from build123d import *

# Parameters (mm, degrees)
F0_R     = 1.5
F0_R_2   = 3
F1_DEPTH = 2


with BuildPart() as f1:
    # F0 (on Top) → F1 (new body)
    with BuildSketch(Plane.XY):
        with BuildLine():
            Line((-31.964893, 11.673815), (-28.487817, 11.673815))
            Line((-28.487817, 11.673815), (-28.487817, 7.80591))
            ThreePointArc((-28.487817, 7.80591), (-24.73358, 5.237709), (-20.981651, 7.80928))
            Line((-20.981651, 7.80928), (-20.981651, 11.050785))
            Line((-20.981651, 11.050785), (-15.487817, 11.050785))
            ThreePointArc((-15.487817, 11.050785), (-13.62272, 14.450413), (-15.487817, 17.850041))
            Line((-15.487817, 17.850041), (-15.487817, 21.423815))
            Line((-15.487817, 21.423815), (-21.987817, 21.423815))
            ThreePointArc((-21.987817, 21.423815), (-24.399065, 23.705329), (-27.288638, 22.071378))
            Line((-27.288638, 22.071378), (-31.889195, 17.850041))
            ThreePointArc((-31.889195, 17.850041), (-33.985999, 17.050288), (-34.987817, 15.042166))
            Line((-34.987817, 15.042166), (-34.987817, 14.481326))
            ThreePointArc((-34.987817, 14.481326), (-34.01389, 12.498791), (-31.964893, 11.673815))
        make_face()
        with Locations((-24.737817, 8.548815)):
            Circle(F0_R, mode=Mode.SUBTRACT)
        with Locations((-32.562817, 14.673815)):
            Circle(F0_R, mode=Mode.SUBTRACT)
        with Locations((-24.737817, 14.673815)):
            Circle(F0_R_2, mode=Mode.SUBTRACT)
        with Locations((-24.737817, 20.798815)):
            Circle(F0_R, mode=Mode.SUBTRACT)
        with Locations((-16.912817, 14.673815)):
            Circle(F0_R, mode=Mode.SUBTRACT)
    extrude(amount=F1_DEPTH)


solid = f1.part
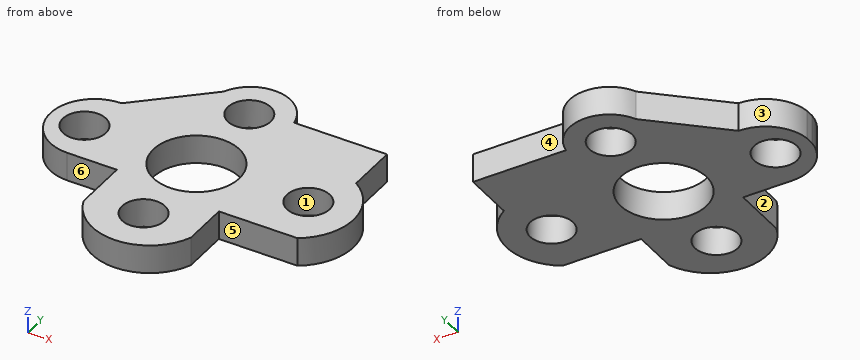
Here's how the part is built. I have some questions about the finished solid (model axes, mm). Face numbers are marked on the shaded views. A direction names the side the tool comes from. Give positions to 0.01 mm unless a question says otherwise; leave off trailing zeros. Loops run counter-clockwise (first coordinate to the right, second up) from the corner with the lowest first, then second, coordinate; pieces in that order, holes last. Notation, with made-up numbers: (84.25, -26) -> (141.25, -26) arc R10 ccw to (141.25, -18) -> close; hole circle Ø5 at (10, 27.25). An arc over 180 degrees is marked (long way). Answer as a JSON object with one key per item and string values. Group by question number.
Item 1: Imagine slicing it at B-B on x = -25.25. Write out the boundary of the cut face in (y, z).
Item 2: Imagine slicing it at D-D on y = 20.25. Write out the boundary of the cut face in (x, z).
Item 3: Imagine slicing it at A-A on y = 15.75. Write out the boundary of the cut face in (x, z), then the cut area to 3 significant figures.
Item 4: Imagine slicing it at C-C on x = -23. Write out the boundary of the cut face in (y, z).
Item 5: I need wall thicknesses on L1, parallel to Y at x = -25, z = 1.2; L2, parallel to X at y = 15.75, z = 0.4; L3, parallel to Y at x = -17.5, z = 0.5. Which ranges of each line are inside material? Lowest first, please.
Item 6: On a 3-axis mill with a long thin cutter (end or side, diameter ignored), from which of +Z, -Z, +X, -X, +Y, -Y can I reach the whole of each face in a straight line? I mean the marked faces 4, 5 and 6. Say none if no direction works.
Item 7: Will these pins go through, and if not, where does the flat tip stop? pin 1 (1 mm diameter, centred on y = 18.5, z = 0.5, fed in from -X); pin 2 (0.6 mm diameter, centred on y = 10.5, z = 1.5, fed in from -X); pin 3 (3.5 mm diameter, centred on x = -24.74, y = 14.67, fed in from +Z); pin 4 (0.6 mm diameter, centred on x = -17, z = 1, fed in from -Y).
Item 8: Thinking about a two-plate mould opening in Y: for the marked faces 1, 2 and 3, which applies, pulls with the +Y half, pulls with the -Y half, needs draft (parallel to the pull), parting line crosses it, or undercut?
Answer list:
{
 "1": {"outline": "(5.27, 0) -> (7.14, 0) -> (7.14, 2) -> (5.27, 2) -> close; (9.96, 0) -> (11.72, 0) -> (11.72, 2) -> (9.96, 2) -> close; (17.63, 0) -> (19.39, 0) -> (19.39, 2) -> (17.63, 2) -> close; (22.21, 0) -> (23.68, 0) -> (23.68, 2) -> (22.21, 2) -> close"},
 "2": {"outline": "(-29.27, 0) -> (-26.13, 0) -> (-26.13, 2) -> (-29.27, 2) -> close; (-23.34, 0) -> (-15.49, 0) -> (-15.49, 2) -> (-23.34, 2) -> close"},
 "3": {"outline": "(-34.84, 0) -> (-33.61, 0) -> (-33.61, 2) -> (-34.84, 2) -> close; (-31.52, 0) -> (-27.54, 0) -> (-27.54, 2) -> (-31.52, 2) -> close; (-21.94, 0) -> (-17.96, 0) -> (-17.96, 2) -> (-21.94, 2) -> close; (-15.87, 0) -> (-13.84, 0) -> (-13.84, 2) -> (-15.87, 2) -> close", "area": "22.4 mm2"},
 "4": {"outline": "(5.63, 0) -> (12.23, 0) -> (12.23, 2) -> (5.63, 2) -> close; (17.12, 0) -> (23.12, 0) -> (23.12, 2) -> (17.12, 2) -> close"},
 "5": {"L1": "y = 5.25 to 7.07, 10.03 to 11.69, 17.66 to 19.32, 22.28 to 23.71", "L2": "x = -34.84 to -33.61, -31.52 to -27.54, -21.94 to -17.96, -15.87 to -13.84", "L3": "y = 11.05 to 13.29, 16.05 to 21.42"},
 "6": {"face 4": "+Z, -Z, +X, +Y", "face 5": "+Z, -Z, +X, -Y", "face 6": "+Z, -Z, -X, -Y"},
 "7": {"pin 1": "stops at x = -31.73", "pin 2": "stops at x = -28.49", "pin 3": "passes through", "pin 4": "stops at y = 11.05"},
 "8": {"face 1": "undercut", "face 2": "needs draft", "face 3": "pulls with the +Y half"}
}
